from build123d import *

# Parameters (mm, degrees)
BOSS_EXTRU_1_DEPTH      = 35.3
ESQUISSE2_W             = 34.2976806
ESQUISSE2_H             = 27.8959906
ENL_V_MAT_EXTRU_1_DEPTH = 34
ENL_V_MAT_EXTRU_5_DEPTH = 34
CONG_1_R                = 0.25
ENL_V_MAT_EXTRU_6_DEPTH = 34
CONG_2_R                = 0.25
BOSS_EXTRU_2_DEPTH      = 2
CHANFREIN1_SIZE         = 1.5
ESQUISSE6_W             = 3.622795385
ESQUISSE6_H             = 7.9
BOSS_EXTRU_4_DEPTH      = 2
CHANFREIN2_SIZE         = 1.5
ESQUISSE7_W             = 7.85
ESQUISSE7_H             = 4.6
ESQUISSE7_H_2           = 4.604428761
BOSS_EXTRU_5_DEPTH      = 2
CHANFREIN3_SIZE         = 1.5


with BuildPart() as part:
    # Esquisse1 → Boss.-Extru.1 (new body)
    with BuildSketch(Plane.XY):
        Polygon((0, 0), (39.5, 0), (39.5, 7.4), (30.9, 7.4), (7.4, 30.9), (7.4, 39.5), (0, 39.5), align=None)
    extrude(amount=-BOSS_EXTRU_1_DEPTH)

    # Esquisse2 → Enlèv. mat.-Extru.1 (cut)
    with BuildSketch(Plane(origin=(0, 39.5, 0), x_dir=(1, 0, 0), z_dir=(0, 1, 0))):
        with Locations((22.3511597, 17.6520047)):
            Rectangle(ESQUISSE2_W, ESQUISSE2_H)
    extrude(amount=-ENL_V_MAT_EXTRU_1_DEPTH, mode=Mode.SUBTRACT)

    # Esquisse3 → Enlèv. mat.-Extru.5 (cut)
    with BuildSketch(Plane(origin=(5.2023194, 0, 0), x_dir=(0, 0, -1), z_dir=(1, 0, 0))):
        with BuildLine():
            Line((18.147028677, 12.354666202), (17.156980723, 12.354666202))
            ThreePointArc((17.156980723, 12.354666202), (14.328553598, 13.526239077), (13.156980723, 16.354666202))
            Line((13.156980723, 16.354666202), (13.156980723, 27.748298541))
            ThreePointArc((13.156980723, 27.748298541), (14.328553598, 30.576725666), (17.156980723, 31.748298541))
            Line((17.156980723, 31.748298541), (18.147028677, 31.748298541))
            ThreePointArc((18.147028677, 31.748298541), (20.975455802, 30.576725666), (22.147028677, 27.748298541))
            Line((22.147028677, 27.748298541), (22.147028677, 16.354666202))
            ThreePointArc((22.147028677, 16.354666202), (20.975455802, 13.526239077), (18.147028677, 12.354666202))
        make_face()
    extrude(amount=-ENL_V_MAT_EXTRU_5_DEPTH, mode=Mode.SUBTRACT)

    # Congé1
    cong_1_edges = [part.edges().sort_by_distance(p)[0] for p in [
        (0, 13.526239077, -20.975455802),
        (0, 12.354666202, -17.6520047),
        (0, 13.526239077, -14.328553598),
        (0, 22.051482371, -13.156980723),
        (0, 30.576725666, -14.328553598),
        (0, 31.748298541, -17.6520047),
        (0, 30.576725666, -20.975455802),
        (0, 22.051482371, -22.147028677),
        (5.2023194, 13.526239077, -20.975455802),
        (5.2023194, 22.051482371, -22.147028677),
        (5.2023194, 30.576725666, -20.975455802),
        (5.2023194, 31.748298541, -17.6520047),
        (5.2023194, 30.576725666, -14.328553598),
        (5.2023194, 22.051482371, -13.156980723),
        (5.2023194, 13.526239077, -14.328553598),
        (5.2023194, 12.354666202, -17.6520047),
    ]]
    fillet(cong_1_edges, radius=CONG_1_R)

    # Esquisse4 → Enlèv. mat.-Extru.6 (cut)
    with BuildSketch(Plane(origin=(0, 5.5, 0), x_dir=(1, 0, 0), z_dir=(0, 1, 0))):
        with BuildLine():
            Line((12.508316826, 17.151207911), (12.508316826, 18.152801489))
            ThreePointArc((12.508316826, 18.152801489), (13.679889701, 20.981228614), (16.508316826, 22.152801489))
            Line((16.508316826, 22.152801489), (27.901153551, 22.152801489))
            ThreePointArc((27.901153551, 22.152801489), (30.729580676, 20.981228614), (31.901153551, 18.152801489))
            Line((31.901153551, 18.152801489), (31.901153551, 17.151207911))
            ThreePointArc((31.901153551, 17.151207911), (30.729580676, 14.322780786), (27.901153551, 13.151207911))
            Line((27.901153551, 13.151207911), (16.508316826, 13.151207911))
            ThreePointArc((16.508316826, 13.151207911), (13.679889701, 14.322780786), (12.508316826, 17.151207911))
        make_face()
    extrude(amount=-ENL_V_MAT_EXTRU_6_DEPTH, mode=Mode.SUBTRACT)

    # Congé2
    cong_2_edges = [part.edges().sort_by_distance(p)[0] for p in [
        (30.729580676, 0, -20.981228614),
        (31.901153551, 0, -17.6520047),
        (30.729580676, 0, -14.322780786),
        (22.204735188, 0, -13.151207911),
        (13.679889701, 0, -14.322780786),
        (12.508316826, 0, -17.6520047),
        (13.679889701, 0, -20.981228614),
        (22.204735188, 0, -22.152801489),
        (30.729580676, 5.5, -20.981228614),
        (22.204735188, 5.5, -22.152801489),
        (13.679889701, 5.5, -20.981228614),
        (12.508316826, 5.5, -17.6520047),
        (13.679889701, 5.5, -14.322780786),
        (22.204735188, 5.5, -13.151207911),
        (30.729580676, 5.5, -14.322780786),
        (31.901153551, 5.5, -17.6520047),
    ]]
    fillet(cong_2_edges, radius=CONG_2_R)

    # Esquisse5 → Boss.-Extru.2 (add)
    with BuildSketch(Plane.XZ):
        Polygon((3.598003918, -17.650224344), (3.598003918, -21.575224344), (7.598003918, -21.575224344), (7.598003918, -17.650473753), (7.598493353, -13.725723193), (3.598493384, -13.725224375), align=None)
    extrude(amount=BOSS_EXTRU_2_DEPTH)

    # Chanfrein1
    chanfrein1_edges = [part.edges().sort_by_distance(p)[0] for p in [
        (7.598248636, -2, -15.688098473),
        (3.598248651, -2, -15.687724359),
        (3.598003918, -2, -19.612724344),
        (7.598003918, -2, -19.612849049),
    ]]
    chamfer(chanfrein1_edges, length=CHANFREIN1_SIZE)

    # Esquisse6 → Boss.-Extru.4 (add)
    with BuildSketch(Plane.XZ):
        with Locations((34.084238676, -17.625224344)):
            Rectangle(ESQUISSE6_W, ESQUISSE6_H)
    extrude(amount=BOSS_EXTRU_4_DEPTH)

    # Chanfrein2
    chanfrein2_edges = [part.edges().sort_by_distance(p)[0] for p in [
        (35.895636368, -2, -17.625224344),
        (32.272840983, -2, -17.625224344),
    ]]
    chamfer(chanfrein2_edges, length=CHANFREIN2_SIZE)

    # Esquisse7 → Boss.-Extru.5 (add)
    with BuildSketch(Plane.ZY):
        with Locations((-17.650224344, 5.512563988)):
            Rectangle(ESQUISSE7_W, ESQUISSE7_H)
        with Locations((-17.650224344, 35.099755073)):
            Rectangle(ESQUISSE7_W, ESQUISSE7_H_2)
    extrude(amount=BOSS_EXTRU_5_DEPTH)

    # Chanfrein3
    chanfrein3_edges = [part.edges().sort_by_distance(p)[0] for p in [
        (-2, 7.812563988, -17.650224344),
        (-2, 3.212563988, -17.650224344),
        (-2, 37.401969453, -17.650224344),
        (-2, 32.797540692, -17.650224344),
    ]]
    chamfer(chanfrein3_edges, length=CHANFREIN3_SIZE)


solid = part.part
Part model, mm, in its own coordinate system. A direction names the side the tool comes from. Round coordinates to 2 decimals unless told otherwise and drop trailing zeros. Order: outer loops, then holes, each group sorted by start corner. A loop starts at its lowest first (then second) coordinate and runs counter-clockwise, first axis right, second up. Notation, with made-up numbers: (22.5, 16.5) -> (71.5, 16.5) arc R15 ccw to (71.5, 41.5) -> close; hole circle Ø3 at (-32, 16). An arc over 180 degrees is marked (long way). Put each result on its own line as item: value.
Q1. Band-saw the part on A-A (y = 26). Give the cut face in (x, z), and give its area (3 significant figures).
From the geometry:
outline: (0, -35.3) -> (12.3, -35.3) -> (12.3, -31.6) -> (5.2, -31.6) -> (5.2, -22.4) arc R0.25 ccw to (4.95, -22.15) -> (0.25, -22.15) arc R0.25 ccw to (0, -22.4) -> close; (0, -12.91) arc R0.25 ccw to (0.25, -13.16) -> (4.95, -13.16) arc R0.25 ccw to (5.2, -12.91) -> (5.2, -3.7) -> (12.3, -3.7) -> (12.3, 0) -> (0, 0) -> close
area: 189 mm2
Q2. Band-saw the part on C-C (z = -1.5). Give the cut face in (x, y).
From the geometry:
outline: (0, 0) -> (39.5, 0) -> (39.5, 7.4) -> (30.9, 7.4) -> (7.4, 30.9) -> (7.4, 39.5) -> (0, 39.5) -> close
Q3. Pull direction Y, two halves, no side cores. Call faces 1 (the face through (22, 5.5, -24)), 2 (the face through (22, 3, -22.153)), 3 (the face through (-1.26, 7.05, -17.71)): pulls with the +Y half, pulls with the -Y half, needs draft (parallel to the pull), parting line crosses it, or undercut.
From the geometry:
face 1: pulls with the +Y half
face 2: needs draft
face 3: undercut
Q4. Band-saw the part on D-D (y = 11.5). Give the cut face in (x, z), and give its area (3 significant figures).
From the geometry:
outline: (0, -35.3) -> (26.8, -35.3) -> (26.8, -31.6) -> (5.2, -31.6) -> (5.2, -3.7) -> (26.8, -3.7) -> (26.8, 0) -> (0, 0) -> close
area: 344 mm2
Q5. Band-saw the part on B-B (x = 22). Give the cut face in (y, z).
From the geometry:
outline: (0, -35.3) -> (16.3, -35.3) -> (16.3, -31.6) -> (5.5, -31.6) -> (5.5, -22.4) arc R0.25 ccw to (5.25, -22.15) -> (0.25, -22.15) arc R0.25 ccw to (0, -22.4) -> close; (0, -12.9) arc R0.25 ccw to (0.25, -13.15) -> (5.25, -13.15) arc R0.25 ccw to (5.5, -12.9) -> (5.5, -3.7) -> (16.3, -3.7) -> (16.3, 0) -> (0, 0) -> close
Q6. Pin check, flat tips, straight feed: pin 1 Ø10 at (x, y) = (30.5, 12) entering from +Z; pin 2 Ø1 at (x, z) = (6, -31) entering from -Y; pin 3 Ø5 at (y, z) = (17.5, -4) entering from -X; pin 4 Ø3 at (x, z) = (34.5, -34) entering from +Y. Stop position of each tip, or through.
From the geometry:
pin 1: stops at z = 0
pin 2: stops at y = 0
pin 3: stops at x = 0
pin 4: stops at y = 7.4
Q7. Tool access for faces 4 (the face through (-1, 5, -21.575)), 5 (the face through (3, 22, -22.147)), 6 (the face through (-1, 5, -13.725)), 7 (the face through (35, 7.4, -2)), 8 (the face through (34, -1, -21.575)): list every direction of +Z, -Z, +X, -X, +Y, -Y with a clear straight run to the whole face (end or side of a thin tool).
From the geometry:
face 4: -Z, -X, +Y, -Y
face 5: +X, -X
face 6: +Z, -X, +Y, -Y
face 7: +Z, -Z, +X, +Y
face 8: -Z, +X, -X, -Y
Q8. Wall check: line 1 (X direction, y = 5, z = -17.5); line 2 (Z direction, x = 25.5, y = 9); line 3 (X direction, y = 11.5, z = -6.5). Give the ranges that are in metal, low to high. Write a range as [from, to].
From the geometry:
line 1: x = [-2, 12.51], [31.9, 39.5]
line 2: z = [-35.3, -31.6], [-3.7, 0]
line 3: x = [0, 5.2]
